Can you work these out from the model? Positions are in its coordinate system, mm. Round coordinates to 2 decimals unless told otherwise and drop trailing zeros. Loops run counter-clockwise (first coordinate to the right, second up) from the corner with the lowest first, then second, coordinate; pieces in that order, holes last.
(1) If I drill on line 1 along Z through (x, y) = (-23, 783.5), over which ranges is the centre line in solid material (lowest first)?
(2) I want a section at A-A on x = -29. Write out the boundary of the cut face in (y, z).
(3) I want a section at C-C on y = 1336. Write out the boundary of the cut face in (x, z), plus the area to 3 significant figures.
(4) I want a section at B-B on z = -22. Write out the boundary of the cut face in (x, y), plus the area to 3 significant figures.
Autodesk Inventor part; units mm, degrees
ref_plane "YZ Plane" through (0, 0, 0) normal (1, 0, 0) x (0, 1, 0)
ref_plane "XZ Plane" through (0, 0, 0) normal (0, 1, 0) x (-1, 0, 0)
ref_plane "XY Plane" through (0, 0, 0) normal (0, 0, 1) x (1, 0, 0)
sketch "Boceto1" plane through (0, 0, 0) normal (0, 1, 0) x (-1, 0, 0)
  line L0 (0, 0) -> (50, 0)
  line L1 (50, 0) -> (50, -50)
  line L2 (50, -50) -> (0, -50)
  line L3 (0, -50) -> (0, 0)
  line L4 (1.5, -48.5) -> (48.5, -48.5)
  line L5 (48.5, -48.5) -> (48.5, -1.5)
  line L6 (48.5, -1.5) -> (1.5, -1.5)
  line L7 (1.5, -1.5) -> (1.5, -48.5)
  line L8 (1.5, -48.5) -> (48.5, -1.5) construction
  line L9 (48.5, -48.5) -> (1.5, -1.5) construction
  point P0 (25, -25)
  dimension "d0" = 50
  dimension "d1" = 50
  dimension "d6" = 1.5
  dimension "d7" = 1.5
  dimension "d8" = 1.5
  dimension "d9" = 1.5
extrude "Extrusión1" add sketch "Boceto1" along normal blind 1681.712
equation "\"d0\" = d1"
equation "\"d7\" = d6"
equation "\"d8\" = d6"
equation "\"d9\" = d6"
properties part number "Mesa_soporte2"
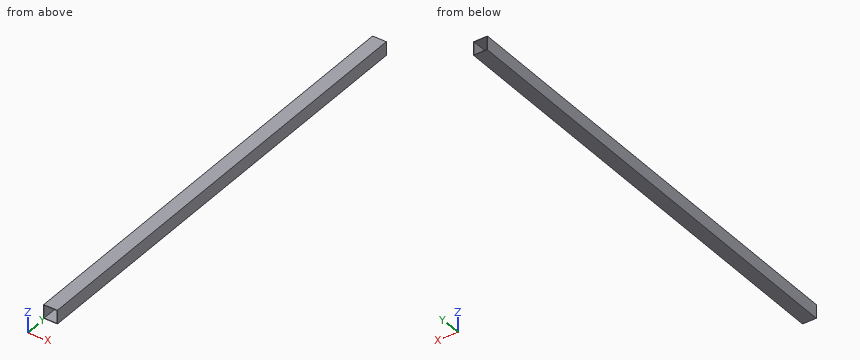
Filled sheet:
1. line 1: z = -50 to -48.5, -1.5 to 0
2. outline: (0, -50) - (1681.71, -50) - (1681.71, -48.5) - (0, -48.5) - close; (0, -1.5) - (1681.71, -1.5) - (1681.71, 0) - (0, 0) - close
3. outline: (-50, -50) - (0, -50) - (0, 0) - (-50, 0) - close; hole (-48.5, -48.5) - (-1.5, -48.5) - (-1.5, -1.5) - (-48.5, -1.5) - close
3. area: 291 mm2
4. outline: (-50, 0) - (-48.5, 0) - (-48.5, 1681.71) - (-50, 1681.71) - close; (-1.5, 0) - (0, 0) - (0, 1681.71) - (-1.5, 1681.71) - close
4. area: 5,050 mm2
